Autodesk Inventor part; units mm, degrees
ref_plane "YZ Plane" through (0, 0, 0) normal (1, 0, 0) x (0, 1, 0)
ref_plane "XZ Plane" through (0, 0, 0) normal (0, 1, 0) x (-1, 0, 0)
ref_plane "XY Plane" through (0, 0, 0) normal (0, 0, 1) x (1, 0, 0)
sketch "Sketch1" plane through (0, 0, 0) normal (0, 1, 0) x (-1, 0, 0)
  point P0 (0, 0)
sketch "Sketch3" plane through (0, 0, 0) normal (0, 1, 0) x (-1, 0, 0)
  circle A0 centre (0, 0) radius 8.2273
  line L0 (0, 0) -> (7.55, 0)
  line L1 (7.55, -2) -> (7.9805, -2)
  line L2 (7.55, 1.9983) -> (7.9813, 1.9967)
  circle A1 centre (-2.7, -1.65) radius 0.6
  line L3 (-2.7, -4.35) -> (-2.7, -4.95)
  circle A2 centre (-2.7, -4.95) radius 0.6
  line L4 (0, -0.6) -> (0, -1.65)
  line L5 (0, -0.6) -> (0, -1.65)
  circle A3 centre (0, 0) radius 0.6
  circle A4 centre (-5.4, -1.65) radius 0.6
  line L6 (-2.7, 1.65) -> (-5.4, 1.65)
  circle A5 centre (-5.4, 1.65) radius 0.6
  line L7 (0, 0.6) -> (0, 3.3)
  circle A6 centre (0, 3.3) radius 0.6
  circle A7 centre (-2.7, 1.65) radius 0.6
  line L8 (-2.7, 1.65) -> (-2.7, 4.95)
  circle A8 centre (-2.7, 4.95) radius 0.6
  line L9 (0, 3.9) -> (0, 6.6)
  circle A9 centre (0, 6.6) radius 0.6
  circle A10 centre (5.4, 0) radius 0.6
  line L10 (2.7, 1.05) -> (2.7, 1.65)
  circle A11 centre (2.7, 1.65) radius 0.6
  line L11 (5.4, 0) -> (5.4, 3.3)
  circle A12 centre (5.4, 3.3) radius 0.6
  line L12 (2.7, 2.25) -> (2.7, 4.95)
  circle A13 centre (2.7, 4.95) radius 0.6
  line L13 (0, -2.7) -> (0, -3.3)
  circle A14 centre (0, -3.3) radius 0.6
  line L14 (0, -3.9) -> (0, -6)
  line L15 (0, -6) -> (0, -6.6)
  circle A15 centre (0, -6.6) radius 0.6
  line L16 (2.7, 0) -> (5.4, 0)
  circle A16 centre (2.7, -1.65) radius 0.6
  line L17 (5.4, 0) -> (5.4, -3.3)
  circle A17 centre (5.4, -3.3) radius 0.6
  line L18 (2.7, -3.75) -> (2.7, -4.95)
  circle A18 centre (2.7, -4.95) radius 0.6
  line L19 (2.7, -1.65) -> (2.7, -3.75)
  line L20 (8.2273, 0.0003) -> (7.0773, 0)
  line L21 (7.0773, 0) -> (7.0773, 2)
  line L22 (7.0773, 2) -> (7.55, 1.9983)
  line L23 (7.0773, 0) -> (7.0773, -2)
  line L24 (7.0773, -2) -> (7.55, -2)
  dimension "d10" = 1.2
  dimension "d15" = 1.2
  dimension "d26" = 1.2
  dimension "d3" = 2
  dimension "d7" = 1.2
  dimension "d8" = 2.1
  dimension "d9" = 0.6
  dimension "d11" = 2.1
  dimension "d12" = 0.6
  dimension "d13" = 1.2
  dimension "d14" = 2.7
  dimension "d16" = 2.7
  dimension "d17" = 1.2
  dimension "d18" = 1.05
  dimension "d20" = 1.2
  dimension "d21" = 2.1
  dimension "d22" = 1.2
  dimension "d23" = 1.2
  dimension "d25" = 0.6
  dimension "d27" = 2.7
  dimension "d28" = 1.2
  dimension "d29" = 2.7
  dimension "d30" = 1.2
  dimension "d31" = 1.2
  dimension "d32" = 1.2
  dimension "d34" = 1.2
  dimension "d35" = 2.7
  dimension "d36" = 0.6
  dimension "d37" = 1.2
  dimension "d38" = 1.2
  dimension "d39" = 1.2
  dimension "d42" = 2.7
  dimension "d46" = 1.15
  dimension "d47" = 2
  dimension "d48" = 2
extrude "Extrusion1" add sketch "Sketch3" along normal blind 3.5 contours L2 L22 L21 L23 L24 L1 A0
properties part number "male"
Work out the finished part from the listing and answer in its coordinate system (mm). A direction names the side the tool comes from. Give positions to 0.01 mm unless a question says otherwise; leave off trailing zeros. Loops run counter-clockwise (first coordinate to the right, second up) from the corner with the lowest first, then second, coordinate; pieces in that order, holes last. Notation, with made-up numbers: (56.25, -27.5) -> (70.25, -27.5) arc R8 ccw to (70.25, -19.5) -> close; hole circle Ø10 at (-5, 1.5). An arc over 180 degrees is marked (long way). Use a Markdown table: item, result. Add a question column.
1) Each of these flat-tipped pins is pushed along its axis until it touches: P1, Ø1, axis at x = -7.5, y = 2.5, coming from the +Z side; P2, Ø1.8, axis at y = 2, z = -0.5, coming from the -X side. Where does it stop, or does it pass through?
2) The part is cut by section C-C, the plane y = 2.05. Count the separate pieces of the cut face and the enclosed holes in it, plus the area to 3 significant figures.
3) The part is cut by section D-D, the plane x = 5.4. Determine the outline of the cut face in (y, z), plus the area to 4 significant figures.
4) For a pull along Z with two mould halves and no side action, classify faces 1 (the cylindrical face through (8.22, 1.73, -0.33)), 2 (the flat face through (-2, 0, 0)), 3 (the flat face through (-7.077, 2, 0)) as +Z half, -Z half, draft (parallel to the pull), parting line (faces both ways), or undercut.
5) Which of the six approach directions +Z, -Z, +X, -X, +Y, -Y give full straight-line access (tool end or side, diameter ignored) to faces 4 (the cylindrical face through (0, 2, -6)), 5 (the flat face through (-7.5, 1.7, -2))?
6) The part is cut by section A-A, the plane x = 0. Determine the outline of the cut face in (y, z).
7) The part is cut by section B-B, the plane z = 0. Determine the outline of the cut face in (x, y), plus the area to 3 significant figures.
8) Consider line 1 along Z through (x, y) = (0, 1.05); line 2 along X through (y, z) = (2.5, 0); line 3 along Z through (x, y) = (-2.7, 2.8). Determine where each line is inside the solid, lowest interval first.
Reported:
| question | item | result |
|---|---|---|
| 1 | P1 | stops at z = 4.32 |
| 1 | P2 | stops at x = -7.08 |
| 2 | separate pieces | 1 |
| 2 | enclosed holes | 18 |
| 2 | area | 188 mm^2 |
| 3 | outline | (0, -6.21) -> (3.5, -6.21) -> (3.5, -2.25) -> (0, -2.25) -> close; (0, -1.05) -> (3.5, -1.05) -> (3.5, 1.05) -> (0, 1.05) -> close; (0, 2.25) -> (3.5, 2.25) -> (3.5, 6.21) -> (0, 6.21) -> close |
| 3 | area | 35.05 mm^2 |
| 4 | face 1 | parting line |
| 4 | face 2 | draft |
| 4 | face 3 | undercut |
| 5 | face 4 | +Y, -Y |
| 5 | face 5 | -X, +Y, -Y |
| 6 | outline | (0, -8.23) -> (3.5, -8.23) -> (3.5, -7.2) -> (0, -7.2) -> close; (0, -6) -> (3.5, -6) -> (3.5, -3.9) -> (0, -3.9) -> close; (0, -2.7) -> (3.5, -2.7) -> (3.5, -0.6) -> (0, -0.6) -> close; (0, 0.6) -> (3.5, 0.6) -> (3.5, 2.7) -> (0, 2.7) -> close; (0, 3.9) -> (3.5, 3.9) -> (3.5, 6) -> (0, 6) -> close; (0, 7.2) -> (3.5, 7.2) -> (3.5, 8.23) -> (0, 8.23) -> close |
| 7 | outline | (-7.08, 0) -> (-6, 0) -> (-6, 3.5) -> (-7.08, 3.5) -> close; (-4.8, 0) -> (-0.6, 0) -> (-0.6, 3.5) -> (-4.8, 3.5) -> close; (0.6, 0) -> (8.23, 0) -> (8.23, 3.5) -> (0.6, 3.5) -> close |
| 7 | area | 45.2 mm^2 |
| 8 | line 1 | z = -8.23 to -7.2, -6 to -3.9, -2.7 to -0.6, 0.6 to 2.7, 3.9 to 6, 7.2 to 8.23 |
| 8 | line 2 | x = -7.08 to -6, -4.8 to -0.6, 0.6 to 8.23 |
| 8 | line 3 | z = -7.77 to -5.55, -4.35 to -2.25, -1.05 to 1.05, 2.25 to 4.35, 5.55 to 7.77 |
